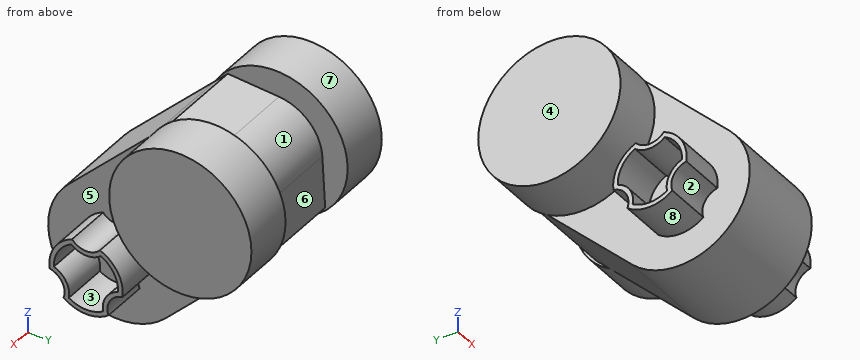
from build123d import *

# Parameters (mm, degrees)
F1_DEPTH = 100
F2_START = 100
F2_DEPTH = 110
F3_DEPTH = 200


with BuildPart() as f1:
    # F0 (on Right) → F1 (new body)
    with BuildSketch(Plane.YZ):
        with BuildLine():
            Line((78.452614635, 290.584648991), (-106.066017178, 106.066017178))
            ThreePointArc((-106.066017178, 106.066017178), (-106.066017178, -106.066017178), (106.066017178, -106.066017178))
            Line((106.066017178, -106.066017178), (290.584648991, 78.452614635))
            ThreePointArc((290.584648991, 78.452614635), (102.530483272, 102.530483272), (78.452614635, 290.584648991))
        make_face()
        with BuildLine():
            ThreePointArc((-79.2845640336, -10.6751068378), (-69.2820323028, 40), (-30.3973683071, 74))
            ThreePointArc((-30.3973683071, 74), (0, 60), (30.3973683071, 74))
            ThreePointArc((30.3973683071, 74), (69.2820323028, 40), (79.2845640336, -10.6751068378))
            ThreePointArc((79.2845640336, -10.6751068378), (51.9615242271, -30), (48.8871957265, -63.3248931622))
            ThreePointArc((48.8871957265, -63.3248931622), (0, -80), (-48.8871957265, -63.3248931622))
            ThreePointArc((-48.8871957265, -63.3248931622), (-51.9615242271, -30), (-79.2845640336, -10.6751068378))
        make_face(mode=Mode.SUBTRACT)
        with BuildLine():
            Line((106.066017178, 318.1980515339), (78.452614635, 290.584648991))
            ThreePointArc((78.452614635, 290.584648991), (102.530483272, 102.530483272), (290.584648991, 78.452614635))
            Line((290.584648991, 78.452614635), (318.1980515339, 106.066017178))
            Line((318.1980515339, 106.066017178), (311.9771141045, 217.6962099463))
            ThreePointArc((311.9771141045, 217.6962099463), (282.8427124746, 282.8427124746), (217.6962099463, 311.9771141045))
            Line((217.6962099463, 311.9771141045), (106.066017178, 318.1980515339))
        make_face()
        with BuildLine():
            ThreePointArc((30.3973683071, 74), (0, 60), (-30.3973683071, 74))
            ThreePointArc((-30.3973683071, 74), (-69.2820323028, 40), (-79.2845640336, -10.6751068378))
            ThreePointArc((-79.2845640336, -10.6751068378), (-51.9615242271, -30), (-48.8871957265, -63.3248931622))
            ThreePointArc((-48.8871957265, -63.3248931622), (0, -80), (48.8871957265, -63.3248931622))
            ThreePointArc((48.8871957265, -63.3248931622), (51.9615242271, -30), (79.2845640336, -10.6751068378))
            ThreePointArc((79.2845640336, -10.6751068378), (69.2820323028, 40), (30.3973683071, 74))
        make_face()
        with BuildLine():
            ThreePointArc((-69.9416518439, -2.8575054411), (-60.6217782649, 35), (-32.4961536185, 62))
            ThreePointArc((-32.4961536185, 62), (0, 50), (32.4961536185, 62))
            ThreePointArc((32.4961536185, 62), (60.6217782649, 35), (69.9416518439, -2.8575054411))
            ThreePointArc((69.9416518439, -2.8575054411), (43.3012701892, -25), (37.4454982254, -59.1424945589))
            ThreePointArc((37.4454982254, -59.1424945589), (0, -70), (-37.4454982254, -59.1424945589))
            ThreePointArc((-37.4454982254, -59.1424945589), (-43.3012701892, -25), (-69.9416518439, -2.8575054411))
        make_face(mode=Mode.SUBTRACT)
        with BuildLine():
            ThreePointArc((32.4961536185, 62), (0, 50), (-32.4961536185, 62))
            ThreePointArc((-32.4961536185, 62), (-60.6217782649, 35), (-69.9416518439, -2.8575054411))
            ThreePointArc((-69.9416518439, -2.8575054411), (-43.3012701892, -25), (-37.4454982254, -59.1424945589))
            ThreePointArc((-37.4454982254, -59.1424945589), (0, -70), (37.4454982254, -59.1424945589))
            ThreePointArc((37.4454982254, -59.1424945589), (43.3012701892, -25), (69.9416518439, -2.8575054411))
            ThreePointArc((69.9416518439, -2.8575054411), (60.6217782649, 35), (32.4961536185, 62))
        make_face()
    extrude(amount=F1_DEPTH)

    # F0 (on Right) → F2 (join)
    with BuildSketch(Plane.YZ.offset(F2_START)):
        with BuildLine():
            Line((106.066017178, 318.1980515339), (78.452614635, 290.584648991))
            ThreePointArc((78.452614635, 290.584648991), (102.530483272, 102.530483272), (290.584648991, 78.452614635))
            Line((290.584648991, 78.452614635), (318.1980515339, 106.066017178))
            Line((318.1980515339, 106.066017178), (311.9771141045, 217.6962099463))
            ThreePointArc((311.9771141045, 217.6962099463), (282.8427124746, 282.8427124746), (217.6962099463, 311.9771141045))
            Line((217.6962099463, 311.9771141045), (106.066017178, 318.1980515339))
        make_face()
        with BuildLine():
            ThreePointArc((367.132034356, 212.132034356), (252.7810807362, 361.7069487914), (78.452614635, 290.584648991))
            Line((78.452614635, 290.584648991), (106.066017178, 318.1980515339))
            Line((106.066017178, 318.1980515339), (217.6962099463, 311.9771141045))
            ThreePointArc((217.6962099463, 311.9771141045), (282.8427124746, 282.8427124746), (311.9771141045, 217.6962099463))
            Line((311.9771141045, 217.6962099463), (318.1980515339, 106.066017178))
            Line((318.1980515339, 106.066017178), (290.584648991, 78.452614635))
            ThreePointArc((290.584648991, 78.452614635), (346.6406869929, 135.1098144075), (367.132034356, 212.132034356))
        make_face()
    extrude(amount=F2_DEPTH)

    # F0 (on Right) → F3 (join)
    with BuildSketch(Plane.YZ):
        with BuildLine():
            ThreePointArc((30.3973683071, 74), (0, 60), (-30.3973683071, 74))
            ThreePointArc((-30.3973683071, 74), (-69.2820323028, 40), (-79.2845640336, -10.6751068378))
            ThreePointArc((-79.2845640336, -10.6751068378), (-51.9615242271, -30), (-48.8871957265, -63.3248931622))
            ThreePointArc((-48.8871957265, -63.3248931622), (0, -80), (48.8871957265, -63.3248931622))
            ThreePointArc((48.8871957265, -63.3248931622), (51.9615242271, -30), (79.2845640336, -10.6751068378))
            ThreePointArc((79.2845640336, -10.6751068378), (69.2820323028, 40), (30.3973683071, 74))
        make_face()
        with BuildLine():
            ThreePointArc((-69.9416518439, -2.8575054411), (-60.6217782649, 35), (-32.4961536185, 62))
            ThreePointArc((-32.4961536185, 62), (0, 50), (32.4961536185, 62))
            ThreePointArc((32.4961536185, 62), (60.6217782649, 35), (69.9416518439, -2.8575054411))
            ThreePointArc((69.9416518439, -2.8575054411), (43.3012701892, -25), (37.4454982254, -59.1424945589))
            ThreePointArc((37.4454982254, -59.1424945589), (0, -70), (-37.4454982254, -59.1424945589))
            ThreePointArc((-37.4454982254, -59.1424945589), (-43.3012701892, -25), (-69.9416518439, -2.8575054411))
        make_face(mode=Mode.SUBTRACT)
    extrude(amount=F3_DEPTH)

    # F4: F1 across face


with BuildPart() as f1_1:
    add(f1.part)
    add(f1.part.mirror(Plane.YZ))


solid = f1_1.part
Build history of the part. All positions in model axes, mm. Face numbers are marked on the shaded views. A direction names the side the tool comes from. Round coordinates to 2 decimals unless told otherwise and drop trailing zeros. Order: outer loops, then holes, each group sorted by start corner. A loop starts at its lowest first (then second) coordinate and runs counter-clockwise, first axis right, second up. Notation, with made-up numbers: M -32.75,-32.5 L 2.25,-32.5 A7 ccw 2.25,-19.5 Z; hole C 75.5,4.5 d10. An arc over 180 degrees is marked long. Use CSV: the item, a comma, the result in double quotes. Start each with the question number.
(1) Flat gauge pins, fed straight in: P1, Ø10, axis at x = -28, z = 260, coming from the +Y side; P2, Ø12, axis at x = -152.5, z = -6, coming from the -Y side; P3, Ø8, axis at x = 9, z = 66, coming from the +Y side. Where does each tip first touch, or does it go through?
(2) Cut at D-D on z = 165. List the corners of the cut face in (x, y).
(3) Cut at C-C on x = -73. List the corners of the cut face in (y, z).
(4) Mould opens along Z. For the marked faces 1, 2, 3 and 4 say: +Z half, -Z half, draft (parallel to the pull), parting line (faces both ways), or undercut.
(5) Cut at A-A on x = -130. List the corners of the cut face in (y, z), then the cut area to 3 significant figures.
(6) Drill centre lines: probe 1 along X at (y, z) = (327, 298); probe 2 along Z at (x, y) = (158.5, -42.5); probe 3 along X at (y, z) = (72, 16). Where is each one in solid material? Low to high.
(7) Cut at B-B on y = 335. List the corners of the cut face in (x, z), then the cut area to 3 significant figures.
(8) Tool access for the marked faces 5, 6, 7 and 8: list every direction of +Z, -Z, +X, -X, +Y, -Y with a clear straight run to the whole face (end or side of a thin tool).
Findings:
1,P1,"stops at y = 302.48"
1,P2,"stops at y = -80"
1,P3,"stops at y = 282.13"
2,outline,"M -210,64.47 L -100,64.47 L -100,-47.13 L 100,-47.13 L 100,64.47 L 210,64.47 L 210,359.79 L 100,359.79 L 100,314.91 L -100,314.91 L -100,359.79 L -210,359.79 Z"
3,outline,"M -106.07,106.07 A150 ccw 106.07,-106.07 L 318.2,106.07 L 311.98,217.7 A100 ccw 217.7,311.98 L 106.07,318.2 Z"
4,face 1,"+Z half"
4,face 2,"undercut"
4,face 3,"undercut"
4,face 4,"draft"
5,outline,"M -79.28,-10.68 A40 cw -48.89,-63.32 A80 ccw 48.89,-63.32 A40 cw 79.28,-10.68 A80 ccw 30.4,74 A40 cw -30.4,74 A80 ccw Z; C 212.13,212.13 d310; hole M -69.94,-2.86 A50 cw -37.45,-59.14 A70 ccw 37.45,-59.14 A50 cw 69.94,-2.86 A70 ccw 32.5,62 A50 cw -32.5,62 A70 ccw Z"
5,area,"80,300 mm^2"
6,probe 1,"x = -210 to -100, 100 to 210"
6,probe 2,"z = -67.78 to -26.44, 55.62 to 67.78"
6,probe 3,"x = -200 to 200"
7,outline,"M -210,117.64 L -100,117.64 L -100,306.62 L -210,306.62 Z; M 100,117.64 L 210,117.64 L 210,306.62 L 100,306.62 Z"
7,area,"41,600 mm^2"
8,face 5,"+X"
8,face 6,"+Z, +Y"
8,face 7,"-X"
8,face 8,"-Z, -X"
